Part print with two shaded views. Sizes in mm from the minimum x, y, z corner. A direction names the side the tool comes from. Round coordinates to 2 decimals unless told otherwise and drop trailing zeros. Loops run counter-clockwise (first coordinate to the right, second up) from the corner with the lowest first, then second, coordinate; pieces in that order, holes last.
(1) Cut at C-C on x = 300. List the corners of the cut face in (y, z), then the cut area to 3 significant figures.
(2) Tool access for the marked faces 4, 5 and 6: list every direction of +Z, -Z, +X, -X, +Y, -Y with a clear straight run to the whole face (end or side of a thin tool).
(3) Cut at A-A on y = 500. List the corners of the cut face in (x, z), then the cut area to 3 significant figures.
(4) Cut at B-B on z = 114. List the corners of the cut face in (x, y), then the cut area to 3 significant figures.
(5) Mould opens along Y. For the marked faces 1, 2 and 3 say: +Y half, -Y half, draft (parallel to the pull), parting line (faces both ways), or undercut.
(6) Cut at D-D on z = 523. List the corners of the cut face in (x, y).
(7) Flat gauge pins, fed straight in: pin 1 (2 mm diameter, centred on x = 331.5, z = 376, fed in from +Y); pin 2 (5 mm diameter, centred on x = 557, z = 479, fed in from -Y). Where does each tip first touch, or does it go through?
(8) Probe probe 1 along Y at (x, z) = (1200, 467); probe 2 along Y at (x, z) = (1091, 134.5); probe 3 along Z at (x, y) = (392, 185.5). List the from-to ranges inside material, lowest first.
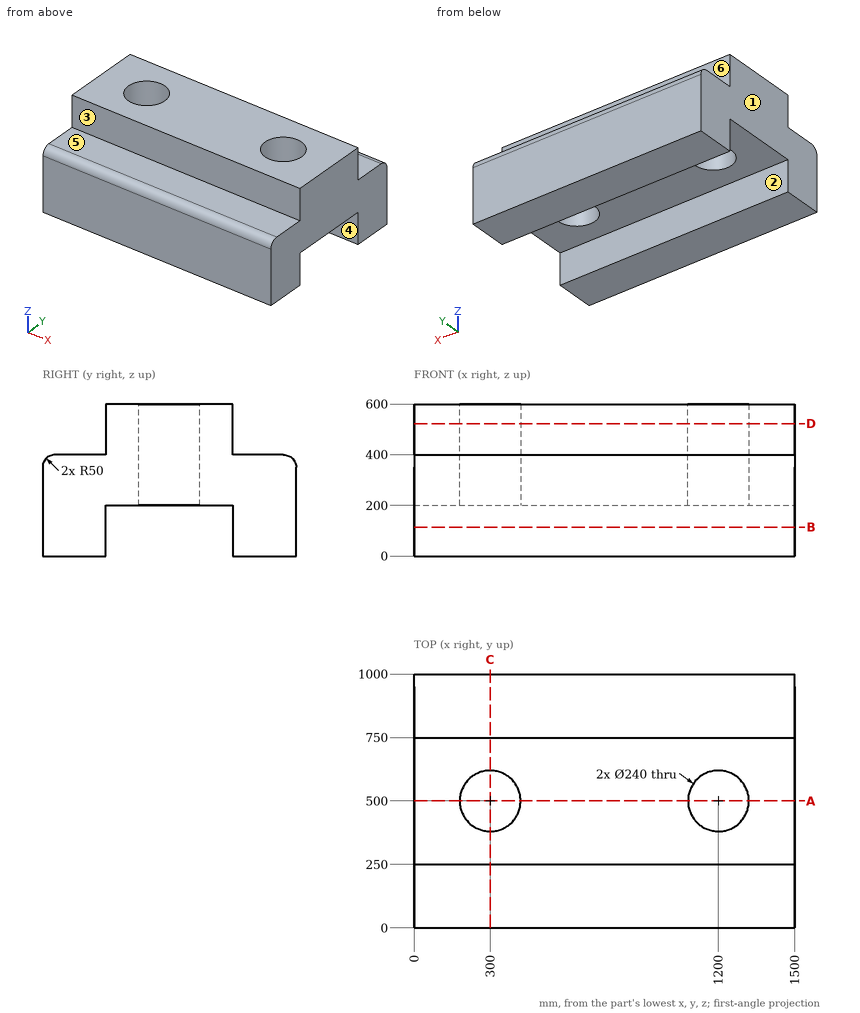
Final values:
1. outline: (0, 0) - (250, 0) - (250, 200) - (380, 200) - (380, 600) - (250, 600) - (250, 400) - (50, 400) arc R50 ccw to (0, 350) - close; (620, 200) - (750, 200) - (750, 0) - (1000, 0) - (1000, 350) arc R50 ccw to (950, 400) - (750, 400) - (750, 600) - (620, 600) - close
1. area: 303,000 mm2
2. face 4: -Z, +X, -X
2. face 5: +Z, +X, -X, -Y
2. face 6: +Z, +X, -X, +Y
3. outline: (0, 200) - (180, 200) - (180, 600) - (0, 600) - close; (420, 200) - (1080, 200) - (1080, 600) - (420, 600) - close; (1320, 200) - (1500, 200) - (1500, 600) - (1320, 600) - close
3. area: 408,000 mm2
4. outline: (0, 0) - (1500, 0) - (1500, 250) - (0, 250) - close; (0, 750) - (1500, 750) - (1500, 1000) - (0, 1000) - close
4. area: 750,000 mm2
5. face 1: draft
5. face 2: undercut
5. face 3: -Y half
6. outline: (0, 250) - (1500, 250) - (1500, 750) - (0, 750) - close; hole circle Ø240 at (300, 500); hole circle Ø240 at (1200, 500)
7. pin 1: stops at y = 993.3
7. pin 2: stops at y = 250
8. probe 1: y = 250 to 380, 620 to 750
8. probe 2: y = 0 to 250, 750 to 1000
8. probe 3: z = 0 to 400
